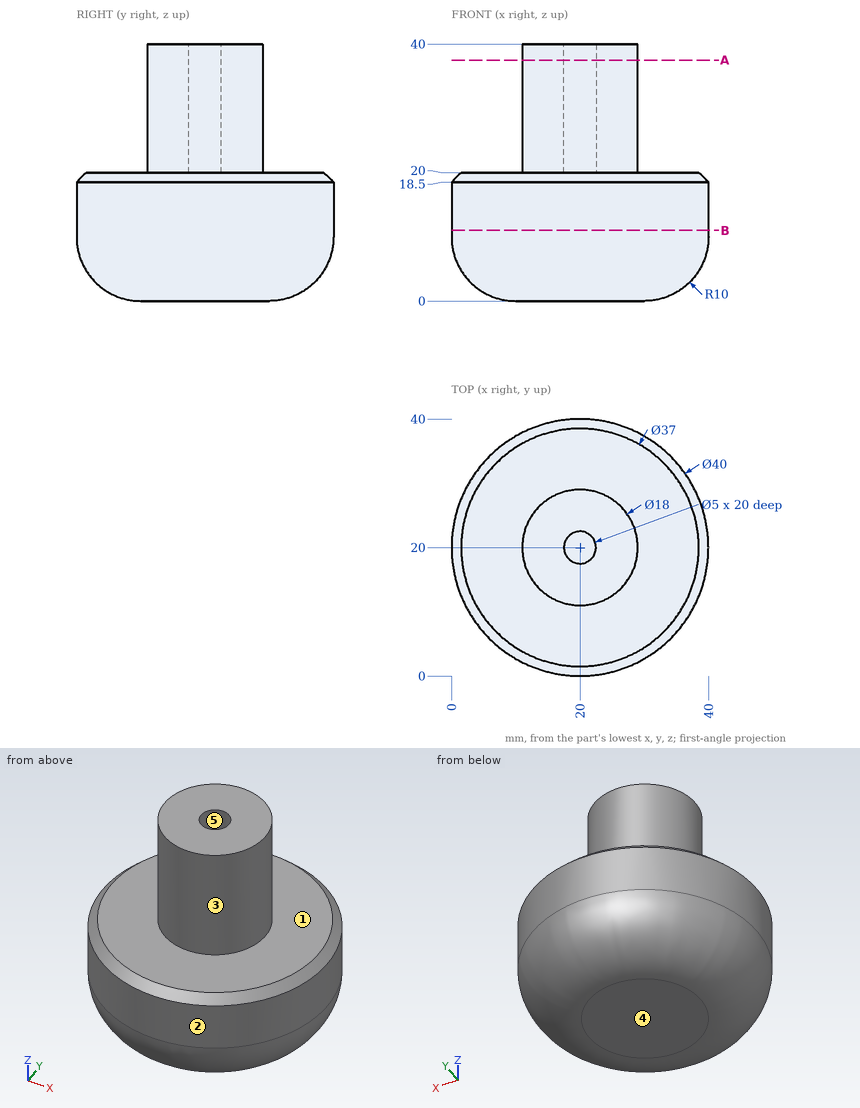
Input: dimensioned drawing with shaded views. Units: mm. Origin: part minimum x, y, z. A direction names the side the tool comes from. Coordinates: 2 decimals unless noted, no trailing zeros. Loops run counter-clockwise (first coordinate to the right, second up) from the corner with the lowest first, then second, coordinate; pieces in that order, holes last. Notation, with made-up numbers: M 11,39.5 L 27,39.5 A9 ccw 27,53.5 Z; hole C 24,63.5 d2. An arc over 180 degrees is marked long. Put each result on its own line as item: value.
(1) Cut plane A-A on z = 37.5. Return the cut outline in (x, y), then the cut area to 3 significant figures.
Answer sheet:
outline: C 20,20 d18; hole C 20,20 d5
area: 235 mm^2
(2) Access query for the marked faces 1 and 2. Directions: +Z, -Z, +X, -X, +Y, -Y. A direction counts if a zero-diameter tool reaches every point of the face in a straight line with its end or side. Return the directions, or none.
Answer sheet:
face 1: +Z
face 2: +Z, -Z
(3) First-contact query: pin 1 (4 mm diameter, centred on x = 15, y = 23.5, fed in from -Z); pin 2 (2 mm diameter, centred on y = 26.5, z = 34, fed in from -X); pin 3 (5 mm diameter, centred on x = 6, y = 16.5, fed in from +Z); pin 4 (3 mm diameter, centred on x = 26.5, y = 33, fed in from -Z). Flat tips, straight axial feed; report the tip coordinate or a pass-through.
Answer sheet:
pin 1: stops at z = 0
pin 2: stops at x = 12.88
pin 3: stops at z = 20
pin 4: stops at z = 0.47
(4) Cut plane B-B on z = 11. Return the cut outline in (x, y), then the cut area to 3 significant figures.
Answer sheet:
outline: C 20,20 d40
area: 1,260 mm^2
(5) Draft query along X for the marked faces 3, 4 and 5. Return one class per face: pulls with the +X half, pulls with the -X half, needs draft (parallel to the pull), parting line crosses it, or undercut.
Answer sheet:
face 3: parting line crosses it
face 4: needs draft
face 5: undercut
(6) Material intervals for probe 1 along Y at (x, z) = (20, 32.5); probe 2 along Z at (x, y) = (18, 38.5); probe 3 along Z at (x, y) = (10.5, 25.5), sorted ascending.
Answer sheet:
probe 1: y = 11 to 17.5, 22.5 to 29
probe 2: z = 4.91 to 19.89
probe 3: z = 0.05 to 20
